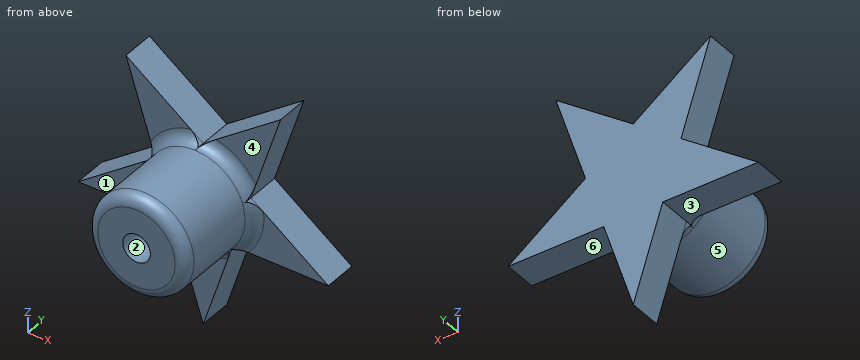
```python
from build123d import *

# Parameters (mm, degrees)
SKETCH2_R                = 4.5
BOSS_EXTRUDE1_DEPTH      = 10
SKETCH4_R                = 1.25
CUT_EXTRUDE1_DEPTH       = 2.5
CUT_EXTRUDE4_DEPTH       = 6
BOSS_EXTRUDE7_DEPTH      = 1.5
BOSS_EXTRUDE7_DEPTH_BACK = 1.5
FILLET2_R                = 1


with BuildPart() as part:
    # Sketch2 → Boss-Extrude1 (new body)
    with BuildSketch(Plane(origin=(0, 0, 0), x_dir=(1, 0, 0), z_dir=(0, 1, 0))):
        with Locations(Location((0, 0, 0), (0, 0, 270))):
            Circle(SKETCH2_R)
    extrude(amount=BOSS_EXTRUDE1_DEPTH)

    # Sketch4 → Cut-Extrude1 (cut)
    with BuildSketch(Plane.XZ):
        with Locations(Location((0, 0, 0), (0, 0, 270))):
            Circle(SKETCH4_R)
    extrude(amount=-CUT_EXTRUDE1_DEPTH, mode=Mode.SUBTRACT)

    # Sketch5 → Cut-Extrude4 (cut)
    with BuildSketch(Plane.XZ.offset(-2.5)):
        with BuildLine():
            Line((-0.75, 1), (-0.75, -1))
            ThreePointArc((-0.75, -1), (0, -1.25), (0.75, -1))
            Line((0.75, -1), (0.75, 1))
            ThreePointArc((0.75, 1), (0, 1.25), (-0.75, 1))
        make_face()
    extrude(amount=-CUT_EXTRUDE4_DEPTH, mode=Mode.SUBTRACT)

    # Sketch3 → Boss-Extrude7 (add, two sides: drawn at the far end of the back side and taken through both)
    with BuildSketch(Plane(origin=(0, 10, 0), x_dir=(1, 0, 0), z_dir=(0, 1, 0)).offset(-BOSS_EXTRUDE7_DEPTH_BACK)):
        Polygon((0, 11.909111317), (-2.673762079, 3.680117785), (-11.326237921, 3.680117785), (-4.326237921, -1.405679911), (-7, -9.634673443), (0, -4.548875747), (7, -9.634673443), (4.326237921, -1.405679911), (11.326237921, 3.680117785), (2.673762079, 3.680117785), align=None)
    extrude(amount=BOSS_EXTRUDE7_DEPTH + BOSS_EXTRUDE7_DEPTH_BACK)

    # Fillet2
    # the kernel refuses this fillet: 1 mm, written as the material it adds along each edge
    with BuildSketch(Plane(origin=(0, 8.5, 0), x_dir=(0, 0, 1), z_dir=(1, 0, 0))) as fillet2_piece_1_section:
        with BuildLine():
            CenterArc((4.5 + FILLET2_R, FILLET2_R), FILLET2_R, 180, 90)
            Line((4.5 + FILLET2_R, 0), (4.5, 0))
            Line((4.5, 0), (4.5, FILLET2_R))
        make_face()
    fillet2_piece_1 = revolve(axis=Axis((0, 8.5, 0), (0, -1, 0)), mode=Mode.PRIVATE)
    fillet2_piece_1 = split(fillet2_piece_1, bisect_by=Plane(origin=(3e-09, 8.080053503, -3.680117785), z_dir=(0, 0, 1)), keep=Keep.TOP, mode=Mode.PRIVATE)
    fillet2_piece_1 = split(fillet2_piece_1, bisect_by=Plane(origin=(-0.015987158, 8.080053503, 4.537260397), z_dir=(0.587785252292471, 0, -0.8090169943749492)), keep=Keep.TOP, mode=Mode.PRIVATE)
    fillet2_piece_1 = split(fillet2_piece_1, bisect_by=Plane(origin=(0.015987161, 8.080053503, 4.537260395), z_dir=(-0.5877852522924681, 0, -0.8090169943749511)), keep=Keep.TOP, mode=Mode.PRIVATE)
    add(fillet2_piece_1)
    with BuildSketch(Plane(origin=(0, 8.5, 0), x_dir=(0, 0, 1), z_dir=(1, 0, 0))) as fillet2_piece_2_section:
        with BuildLine():
            CenterArc((4.5 + FILLET2_R, FILLET2_R), FILLET2_R, 180, 90)
            Line((4.5 + FILLET2_R, 0), (4.5, 0))
            Line((4.5, 0), (4.5, FILLET2_R))
        make_face()
    fillet2_piece_2 = revolve(axis=Axis((0, 8.5, 0), (0, -1, 0)), mode=Mode.PRIVATE)
    fillet2_piece_2 = split(fillet2_piece_2, bisect_by=Plane(origin=(-4.906405348, 8.214560611, 3.191251651), z_dir=(0.9510565162951518, 0, 0.30901699437495306)), keep=Keep.TOP, mode=Mode.PRIVATE)
    fillet2_piece_2 = split(fillet2_piece_2, bisect_by=Plane(origin=(4.369206305, 8.214560611, 1.537922999), z_dir=(-0.9510565162951523, 0, 0.30901699437495134)), keep=Keep.TOP, mode=Mode.PRIVATE)
    fillet2_piece_2 = split(fillet2_piece_2, bisect_by=Plane(origin=(-1.518898049, 8.214560611, 5.652419775), z_dir=(-0.5877852522924681, 0, -0.8090169943749511)), keep=Keep.TOP, mode=Mode.PRIVATE)
    add(fillet2_piece_2)
    with BuildSketch(Plane(origin=(0, 8.5, 0), x_dir=(0, 0, 1), z_dir=(1, 0, 0))) as fillet2_piece_3_section:
        with BuildLine():
            CenterArc((4.5 + FILLET2_R, FILLET2_R), FILLET2_R, 180, 90)
            Line((4.5 + FILLET2_R, 0), (4.5, 0))
            Line((4.5, 0), (4.5, FILLET2_R))
        make_face()
    fillet2_piece_3 = revolve(axis=Axis((0, 8.5, 0), (0, -1, 0)), mode=Mode.PRIVATE)
    fillet2_piece_3 = split(fillet2_piece_3, bisect_by=Plane(origin=(4.906405349, 8.214560608, 3.191251652), z_dir=(-0.9510565162951523, 0, 0.30901699437495134)), keep=Keep.TOP, mode=Mode.PRIVATE)
    fillet2_piece_3 = split(fillet2_piece_3, bisect_by=Plane(origin=(1.51889805, 8.214560608, 5.652419777), z_dir=(0.587785252292471, 0, -0.8090169943749492)), keep=Keep.TOP, mode=Mode.PRIVATE)
    fillet2_piece_3 = split(fillet2_piece_3, bisect_by=Plane(origin=(2.163118969, 8.214560608, 2.977277823), z_dir=(0.5877852522924681, 0, 0.8090169943749511)), keep=Keep.TOP, mode=Mode.PRIVATE)
    add(fillet2_piece_3)
    # the kernel refuses this fillet: 1 mm, written as the material it takes off along each edge
    with BuildSketch(Plane(origin=(0, 0, 0), x_dir=(0, 0, 1), z_dir=(-1, 0, 0))) as fillet2_2_piece_1:
        with BuildLine():
            CenterArc((4.5 - FILLET2_R, FILLET2_R), FILLET2_R, 270, 90)
            Line((4.5 - FILLET2_R, 0), (4.5, 0))
            Line((4.5, 0), (4.5, FILLET2_R))
        make_face()
    revolve(axis=Axis((0, 0, 0), (0, 1, 0)), mode=Mode.SUBTRACT)


solid = part.part
```
Work out the finished part from the listing and answer in its coordinate system (mm). Face numbers are marked on the shaded views. A direction names the side the tool comes from. Coordinates: 2 decimals unless noted, no trailing zeros. Write each loop counter-clockwise with the first axis right and the second up, starting at its lowest first coordinate (ties: lowest second). Pieces come first, ordered by that corner, then holes. Notation, with made-up numbers: (35, 63) - (54, 63) arc R30 cw to (54, 88) - close; hole circle Ø5 at (88.25, 88.25). An arc over 180 degrees is marked (long way). Answer as a JSON object with one key per item and string values.
Q1. Which of the six approach directions +Z, -Z, +X, -X, +Y, -Y give full straight-line access (tool end or side, diameter ignored) to the marked faces 4, 5 and 6?
Results list:
{"face 4": "+Z, +X, -Y", "face 5": "-Y", "face 6": "-Z, +X, +Y, -Y"}
Q2. Find section A-A (y = 5.75). Write down the section's boundary in (x, z).
Results list:
{"outline": "circle Ø9 at (0, 0); hole (-0.75, -1) arc R1.25 ccw to (0.75, -1) - (0.75, 1) arc R1.25 ccw to (-0.75, 1) - close"}
Q3. Consider L1, parallel to Z at x = 0, y = 4; L2, parallel to X at y = 5, z = 0; L3, parallel to X at y = 11, z = 4.75. Determine where each line is inside the solid, lowest interval first. Write a range as from..to.
Results list:
{"L1": "z = -4.5..-1.25, 1.25..4.5", "L2": "x = -4.5..-0.75, 0.75..4.5", "L3": "x = -5.41..-0.28, 0.28..5.41"}
Q4. For a pull along Z with two mould halves and no side action, classify the marked faces 1, 2 and 3 as pulls with the +Z half, pulls with the -Z half, needs draft (parallel to the pull), parting line crosses it, or undercut.
Results list:
{"face 1": "needs draft", "face 2": "undercut", "face 3": "pulls with the -Z half"}
Q5. Find section C-C (z = -6.75). Write down the section's boundary in (x, y).
Results list:
{"outline": "(-1.68, 8.5) - (1.68, 8.5) - (1.68, 11.5) - (-1.68, 11.5) - close"}
Q6. Given pin 1 Ø1.2 at (x, z) = (0, 0.5) entering from -Y; pin 2 Ø4 at (x, y) = (5, 10) entering from -Z; pin 3 Ø1.5 at (y, z) = (7.5, -7) entering from -X; pin 4 Ø5 at (x, z) = (0, -7.5) entering from -Y, each flat-ended and moving along its own axis, determine where each tip first touches the part or whether it passes through.
Results list:
{"pin 1": "stops at y = 8.5", "pin 2": "stops at z = -3.68", "pin 3": "passes through", "pin 4": "stops at y = 8.37"}
Q7. Find section B-B (z = 0). Write down the section's boundary in (x, y), plus the area to 3 significant figures.
Results list:
{"outline": "(-6.26, 8.5) - (-5.5, 8.5) arc R1 cw to (-4.5, 7.5) - (-4.5, 1) arc R1 ccw to (-3.5, 0) - (-1.25, 0) - (-1.25, 2.5) - (-0.75, 2.5) - (-0.75, 8.5) - (0.75, 8.5) - (0.75, 2.5) - (1.25, 2.5) - (1.25, 0) - (3.5, 0) arc R1 ccw to (4.5, 1) - (4.5, 7.5) arc R1 cw to (5.5, 8.5) - (6.26, 8.5) - (6.26, 11.5) - (-6.26, 11.5) - close", "area": "98.8 mm^2"}
